Geometry check sheet. Reference: the model listing, model coordinates, mm. A direction names the side the tool comes from. Give positions to 0.01 mm unless a question says otherwise; leave off trailing zeros. Write each loop counter-clockwise with the first axis right and the second up, starting at its lowest first coordinate (ties: lowest second). Pieces come first, ordered by that corner, then holes.
(1) Thickness scan on line 1 along X through (y, z) = (-4, 18.25); line 2 along Z through (x, y) = (6.5, 0); line 3 along Y through (x, z) = (-8.5, 15.75). Record the ranges inside material, lowest first.
(2) Mould release check, pull along X, two halves, no side actions. Record for faces 1 (the flat face through (-3.59, 0, 14)), 2 (the cylindrical face through (-9.43, 11.697, 7.395)), 3 (the flat face through (3.51, 0, 14)), 4 (the cylindrical face through (5.79, 9.45, 21.99)): +X half, -X half, draft (parallel to the pull), parting line (faces both ways), or undercut.
(3) Depth check by flat-ended pin: P1, Ø12, axis at x = -7.5, z = 22, coming from the +Y side; P2, Ø3.5, axis at x = -0.5, y = 0.5, coming from the +Z side; P3, Ø4, axis at x = 7, y = 8, coming from the +Z side; P4, Ø2.5, axis at y = 0, z = 16.93, coming from the -X side (3 decimals). Enter the tip coordinate at first touch or a pass-through.
(4) Cross-section at A-A (y = 0). Record the boundary of the cut face in (x, z), and give its area (3 significant figures).
(5) Cross-section at D-D (x = 1.75). Record the boundary of the cut face in (y, z), and give its area (3 significant figures).
(6) Cross-section at B-B (z = 7.75). Record the boundary of the cut face in (x, y).
(7) Tool access check on faces 5 (the flat face through (0, 12.299, 6)), 6 (the flat face through (0, 0, 6.5)). Record the directions out of +Z, -Z, +X, -X, +Y, -Y that give a thin tool (end or side, any length) a straight path to the whole face; none if there is none.
(8) Cross-section at C-C (x = -5.5). Record the boundary of the cut face in (y, z).
```python
from build123d import *

# Parameters (mm, degrees)
F0_W     = 20
F0_H     = 24.5975396182
F1_DEPTH = 25
F2_W     = 7.1
F2_H     = 19.9254054902
F3_DEPTH = 12.5
F4_R     = 2
F5_DEPTH = 20.001
F6_R     = 10
F7_R     = 2
F8_R     = 2


with BuildPart() as f1:
    # F0 (on Top) → F1 (new body)
    with BuildSketch(Plane.XY):
        Rectangle(F0_W, F0_H)
    extrude(amount=F1_DEPTH)

    # F2 (on Front) → F3 (cut, symmetric)
    with BuildSketch(Plane.XZ):
        with Locations((-0.04, 16.4627027451)):
            Rectangle(F2_W, F2_H)
    extrude(amount=F3_DEPTH, both=True, mode=Mode.SUBTRACT)

    # F4 (on face) → F5 (cut, through all)
    with BuildSketch(Plane.YZ.offset(10)):
        with Locations((0, 16.9262466765)):
            Circle(F4_R)
    extrude(amount=-F5_DEPTH, mode=Mode.SUBTRACT)

    # F6
    f6_edges = [f1.edges().sort_by_distance(p)[0] for p in [
        (-6.795, -12.29877, 25),
        (6.755, -12.29877, 25),
        (6.755, 12.29877, 25),
        (-6.795, 12.29877, 25),
    ]]
    fillet(f6_edges, radius=F6_R)

    # F7
    f7_edges = [f1.edges().sort_by_distance(p)[0] for p in [
        (10, -9.369838, 22.071068),
        (10, 0, 25),
    ]]
    fillet(f7_edges, radius=F7_R)

    # F8
    f8_edges = [f1.edges().sort_by_distance(p)[0] for p in [
        (-10, 9.369838, 22.071068),
    ]]
    fillet(f8_edges, radius=F8_R)


solid = f1.part
```
Reply:
1. line 1: x = -10 to -3.59, 3.51 to 10
1. line 2: z = 0 to 14.93, 18.93 to 25
1. line 3: y = -12.21 to -1.62, 1.62 to 12.21
2. face 1: undercut
2. face 2: -X half
2. face 3: undercut
2. face 4: draft
3. P1: stops at y = 12.25
3. P2: stops at z = 6.5
3. P3: stops at z = 24.29
3. P4: passes through
4. outline: (-10, 0) - (10, 0) - (10, 14.93) - (3.51, 14.93) - (3.51, 6.5) - (-3.59, 6.5) - (-3.59, 14.93) - (-10, 14.93) - close; (-10, 18.93) - (-3.59, 18.93) - (-3.59, 25) - (-8, 25) arc R2 ccw to (-10, 23) - close; (3.51, 18.93) - (10, 18.93) - (10, 23) arc R2 ccw to (8, 25) - (3.51, 25) - close
4. area: 315 mm2
5. outline: (-12.3, 0) - (12.3, 0) - (12.3, 6.5) - (-12.3, 6.5) - close
5. area: 160 mm2
6. outline: (-10, -10.3) arc R2 ccw to (-8, -12.3) - (-3.59, -12.3) - (-3.59, 12.3) - (-8, 12.3) arc R2 ccw to (-10, 10.3) - close; (3.51, -12.3) - (8, -12.3) arc R2 ccw to (10, -10.3) - (10, 10.3) arc R2 ccw to (8, 12.3) - (3.51, 12.3) - close
7. face 5: +Z, -Z, +X, -X, +Y
7. face 6: +Z, +Y, -Y
8. outline: (-12.3, 0) - (12.3, 0) - (12.3, 15) arc R10 ccw to (2.3, 25) - (-2.3, 25) arc R10 ccw to (-12.3, 15) - close; hole circle Ø4 at (0, 16.93)
